Autodesk Inventor part; units mm, degrees
ref_plane "YZ Plane" through (0, 0, 0) normal (1, 0, 0) x (0, 1, 0)
ref_plane "XZ Plane" through (0, 0, 0) normal (0, 1, 0) x (-1, 0, 0)
ref_plane "XY Plane" through (0, 0, 0) normal (0, 0, 1) x (1, 0, 0)
sketch "Sketch1" plane through (0, 0, 0) normal (0, 1, 0) x (-1, 0, 0)
  line L0 (119.875, 68.5) -> (-154.125, 68.5)
  line L1 (-154.125, 68.5) -> (-154.125, 8.5)
  line L2 (-154.125, 8.5) -> (119.875, 8.5)
  line L3 (119.875, 8.5) -> (119.875, 68.5)
  point P0 (0, 0)
  dimension "d0" = 274
  dimension "d1" = 60
extrude "Extrusion1" add sketch "Sketch1" along normal blind 10
sketch "Sketch2" plane through (0, 10, 0) normal (0, 1, 0) x (1, 0, 0)
  line L0 (-119.875, -8.5) -> (-119.875, -68.5)
  line L1 (-119.875, -68.5) -> (154.125, -68.5)
  line L2 (154.125, -68.5) -> (154.125, -53.5)
  line L3 (154.125, -53.5) -> (-119.875, -53.5)
  line L4 (-119.875, -53.5) -> (-119.875, -68.5)
  line L5 (154.125, -68.5) -> (154.125, -8.5)
  line L6 (154.125, -8.5) -> (-119.875, -8.5)
  line L7 (-119.875, -8.5) -> (-119.875, -68.5)
  line L8 (-119.875, -68.5) -> (154.125, -68.5)
  point P0 (0, 0)
  dimension "d4" = 15
extrude "Extrusion2" add sketch "Sketch2" along normal blind 50 contours L3 L2 L1 L0
sketch "Sketch3" plane through (0, 10, 0) normal (0, 1, 0) x (1, 0, 0)
  line L0 (154.125, -8.5) -> (108.625, -8.5)
  line L1 (108.625, -8.5) -> (108.625, -54)
  line L2 (108.625, -54) -> (154.125, -54)
  line L3 (154.125, -54) -> (154.125, -8.5)
  line L4 (-119.875, -8.5) -> (-119.875, -68.5)
  line L5 (-119.875, -8.5) -> (-74.375, -8.5)
  line L6 (-74.375, -8.5) -> (-74.375, -54)
  line L7 (-74.375, -54) -> (-119.875, -54)
  line L8 (-119.875, -54) -> (-119.875, -8.5)
  point P0 (0, 0)
  dimension "d7" = 45.5
  dimension "d8" = 45.5
extrude "Extrusion3" cut sketch "Sketch3" along normal mid plane 150
sketch "Sketch4" plane through (0, 0, 0) normal (0, -1, 0) x (1, 0, 0)
  line L0 (-74.375, 54) -> (-74.375, 8.5)
  line L1 (108.625, 8.5) -> (-74.375, 8.5)
  line L2 (108.625, 8.5) -> (108.625, 54)
  line L3 (108.625, 54) -> (154.125, 54)
  line L4 (154.125, 68.5) -> (154.125, 54)
  line L5 (-119.875, 68.5) -> (154.125, 68.5)
  line L6 (-119.875, 54) -> (-119.875, 68.5)
  line L7 (-119.875, 54) -> (-74.375, 54)
  line L8 (-119.875, 68.5) -> (-134.875, 68.5)
  line L9 (-134.875, 68.5) -> (-134.875, 8.5)
  line L10 (-134.875, 8.5) -> (-119.875, 8.5)
  line L11 (-119.875, 8.5) -> (-119.875, 68.5)
  line L12 (154.125, 68.5) -> (169.125, 68.5)
  line L13 (169.125, 68.5) -> (169.125, 8.5)
  line L14 (169.125, 8.5) -> (154.125, 8.5)
  line L15 (154.125, 8.5) -> (154.125, 68.5)
  point P0 (0, 0)
  dimension "d11" = 60
  dimension "d12" = 60
  dimension "d13" = 15
  dimension "d14" = 15
extrude "Extrusion4" add sketch "Sketch4" against normal blind 50 contours L11 L10 L9 L8 L6 | L12 L13 L14 L15 L4
sketch "Sketch5" plane through (0, 60, 0) normal (0, 1, 0) x (1, 0, 0)
  line L0 (-140, -80) -> (185, -80)
  line L1 (185, -80) -> (185, 19)
  line L2 (185, 19) -> (-140, 19)
  line L3 (-140, 19) -> (-140, -80)
  point P0 (0, 0)
extrude "Extrusion5" cut sketch "Sketch5" against normal up to surface (10 mm away)
properties part number "VerticalAxis"
Input: part model. Units: mm. Frame: model coordinates. A direction names the side the tool comes from. Give positions to 0.01 mm unless a question says otherwise; leave off trailing zeros. Order: outer loops, then holes, each group sorted by start corner. A loop starts at its lowest first (then second) coordinate and runs counter-clockwise, first axis right, second up. Notation, with made-up numbers: M 3,5.5 L 26,5.5 A19 ccw 26,18.5 Z; hole C 55.5,-27 d2. An arc over 180 degrees is marked long. One line per question, with ' | ' between items.
1) Section B-B on y = 5.5. Output: boundary loops of the cut face in (x, z) (3 decimals), and give its area (3 significant figures).
Filled in:
outline: M -134.875,8.5 L -119.875,8.5 L -119.875,54 L -74.375,54 L -74.375,8.5 L 108.625,8.5 L 108.625,54 L 154.125,54 L 154.125,8.5 L 169.125,8.5 L 169.125,68.5 L -134.875,68.5 Z | area: 14,100 mm2
2) Ray query, L1, parallel to X at y = 2, z = 28.5 (3 decimals); L2, parallel to X at y = 46.5, z = 16.5 (3 decimals); L3, parallel to Z at x = 79.5, y = 23. Return the intervals inside material, ascending.
Filled in:
L1: x = -134.875 to -119.875, -74.375 to 108.625, 154.125 to 169.125 | L2: x = -134.875 to -119.875, 154.125 to 169.125 | L3: z = 53.5 to 68.5
3) Access query for faces 4 (the face through (-119.875, 25, 31)), 5 (the face through (16, 50, 56)), 6 (the face through (18, 30, 53.5)). Directions: +Z, -Z, +X, -X, +Y, -Y. A direction counts if a zero-diameter tool reaches every point of the face in a straight line with its end or side. Return the directions, or none.
Filled in:
face 4: -Z, +Y, -Y | face 5: +Z, -Z, +X, -X, +Y | face 6: -Z, +Y
4) Section C-C on x = 42. Output: boundary loops of the cut face in (y, z), and give its area (3 significant figures).
Filled in:
outline: M 0,8.5 L 10,8.5 L 10,53.5 L 50,53.5 L 50,68.5 L 0,68.5 Z | area: 1,200 mm2
5) Section D-D on y = 22.5. Output: boundary loops of the cut face in (x, z) (3 decimals).
Filled in:
outline: M -134.875,8.5 L -119.875,8.5 L -119.875,54 L -74.375,54 L -74.375,53.5 L 108.625,53.5 L 108.625,54 L 154.125,54 L 154.125,8.5 L 169.125,8.5 L 169.125,68.5 L -134.875,68.5 Z
6) Draft query along X for faces 1 (the face through (169.125, 25, 39)), 2 (the face through (162, 25, 8.5)), 3 (the face through (108.625, 5, 31)). Return one class per face: pulls with the +X half, pulls with the -X half, needs draft (parallel to the pull), parting line crosses it, or undercut.
Filled in:
face 1: pulls with the +X half | face 2: needs draft | face 3: undercut
7) Contact query for flat-ended pins moving along their axis: P1, Ø1.5, axis at x = 67.5, z = 52.5, coming from the +Y side; P2, Ø2, axis at x = 102.5, y = 41, coming from the -Z side; P3, Ø13.5, axis at x = 127.5, y = 18.5, coming from the -Z side. Output: stop coordinate, or through.
Filled in:
P1: stops at y = 10 | P2: stops at z = 53.5 | P3: stops at z = 54
8) Section A-A on z = 40. Output: boundary loops of the cut face in (x, y) (3 decimals).
Filled in:
outline: M -134.875,0 L -119.875,0 L -119.875,50 L -134.875,50 Z; M -74.375,0 L 108.625,0 L 108.625,10 L -74.375,10 Z; M 154.125,0 L 169.125,0 L 169.125,50 L 154.125,50 Z
